Source: CAD feature listing. Evaluate the final solid. Frame: model axes, mm. Face numbers are marked on the shaded views. A direction names the side the tool comes from. Round coordinates to 2 decimals unless told otherwise and drop trailing zeros. Write each loop counter-clockwise with the first axis right and the second up, starting at its lowest first coordinate (ties: lowest second). Pieces come first, ordered by that corner, then holes.
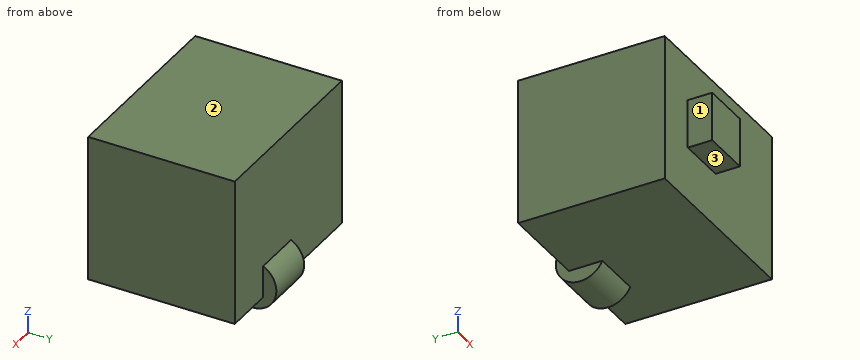
from build123d import *

# Parameters (mm, degrees)
F0_W       = 76.2
F0_H       = 76.2
F1_DEPTH   = 76.2
F2_W       = 25.4
F2_H       = 25.4
F3_DEPTH   = 12.7
F4_R       = 12.7
F1_FACE1_W = 76.2
F1_FACE1_H = 76.2
F5_DEPTH   = 21.59
F6_DEPTH   = 25.4


with BuildPart() as f1:
    # F0 (on Front) → F1 (new body)
    with BuildSketch(Plane.XZ):
        with Locations((-15.8040157244, 72.1577832595)):
            Rectangle(F0_W, F0_H)
    extrude(amount=F1_DEPTH)

    # F2 (on face) → F3 (join)
    with BuildSketch(Plane.XZ.offset(76.2)):
        with Locations((-20.2220443964, 74.8119402349)):
            Rectangle(F2_W, F2_H)
    extrude(amount=F3_DEPTH)

    # F4 (on face) + F1_face1 (on face) → F5 (join)
    with BuildSketch(Plane.YZ.offset(-7.5220443964)):
        with Locations((-5.8702160604, 39.4294373691)):
            Circle(F4_R)
    with BuildSketch(Plane(origin=(22.2959842756, -38.1, 72.1577832595), x_dir=(0, 1, 0), z_dir=(1, 0, 0))):
        Rectangle(F1_FACE1_W, F1_FACE1_H)
    extrude(amount=F5_DEPTH)

    # F4 (on face) → F6 (join)
    with BuildSketch(Plane.YZ.offset(-7.5220443964)):
        with Locations((-5.8702160604, 39.4294373691)):
            Circle(F4_R)
    extrude(amount=F6_DEPTH)


solid = f1.part
1) Contact query for flat-ended pins moving along their axis: P1, Ø10, axis at y = -85, z = 73, coming from the +X side; P2, Ø23, axis at x = 6, y = -43.5, coming from the -Z side; P3, Ø14, axis at y = -84.5, z = 81, coming from the -X side. Output: stop coordinate, or through.
Taken from the geometry:
P1: stops at x = -7.52
P2: stops at z = 34.06
P3: stops at x = -32.92
2) Material intervals for line 1 (Z direction, x = -23.5, y = -1); line 2 (X direction, y = -76.5, z = 84.5); line 3 (Y direction, x = -16, z = 41), sorted ascending.
Taken from the geometry:
line 1: z = 34.06 to 110.26
line 2: x = -32.92 to -7.52
line 3: y = -76.2 to 0
3) Section query C-C on y = -58. Return the cut outline in (x, z).
Taken from the geometry:
outline: (-53.9, 34.06) - (43.89, 34.06) - (43.89, 110.26) - (-53.9, 110.26) - close
4) Reachability of the marked faces 1, 2 and 3 from +Z, -Z, +X, -X, +Y, -Y: full face, straight path, thin tool, end or side. Return the list, or none.
Taken from the geometry:
face 1: +Z, -Z, -X, -Y
face 2: +Z, +X, -X, +Y, -Y
face 3: -Z, +X, -X, -Y
5) Section query D-D on x = -39.5. Return the cut outline in (y, z).
Taken from the geometry:
outline: (-76.2, 34.06) - (0, 34.06) - (0, 110.26) - (-76.2, 110.26) - close
6) Section query A-A on z = 80.5. Return the cut outline in (x, y), then the cut area to 3 significant figures.
Taken from the geometry:
outline: (-53.9, -76.2) - (-32.92, -76.2) - (-32.92, -88.9) - (-7.52, -88.9) - (-7.52, -76.2) - (43.89, -76.2) - (43.89, 0) - (-53.9, 0) - close
area: 7,770 mm2
7) Section query B-B on x = -10. Return the cut outline in (y, z).
Taken from the geometry:
outline: (-88.9, 62.11) - (-76.2, 62.11) - (-76.2, 34.06) - (0, 34.06) - (0, 110.26) - (-76.2, 110.26) - (-76.2, 87.51) - (-88.9, 87.51) - close
